```python
from build123d import *

# Parameters (mm, degrees)
F0_W      = 38.1
F0_H      = 38.1
F0_R      = 6.746875
F1_DEPTH  = 95.25
F3_D      = 4.0386
F3_DEPTH  = 12.7
F3_TIP    = 1.213317848
F5_D      = 4.0386
F5_DEPTH  = 12.7
F5_TIP    = 1.213317848
F6_R      = 9.525
F6_R_2    = 6.746875
F7_DEPTH  = 2.921
F8_R      = 9.525
F8_R_2    = 6.746875
F9_DEPTH  = 2.921
F11_D     = 8.45058
F11_DEPTH = 15.875
F11_TIP   = 2.538810365


with BuildPart() as f1:
    # F0 (on Front) → F1 (new body)
    with BuildSketch(Plane.XZ):
        Rectangle(F0_W, F0_H)
        Circle(F0_R, mode=Mode.SUBTRACT)
    extrude(amount=F1_DEPTH)

    # F3
    with Locations(Plane(origin=(0, 0, 0), x_dir=(-1, 0, 0), z_dir=(0, 1, 0))):
        with Locations((-12.7, -12.7), (-12.7, 12.7), (12.7, 12.7), (12.7, -12.7)):
            Hole(F3_D / 2, depth=F3_DEPTH)
            with Locations((0, 0, -(F3_DEPTH + F3_TIP / 2))):  # 118° drill point
                Cone(0, F3_D / 2, F3_TIP, mode=Mode.SUBTRACT)

    # F5
    with Locations(Plane.XZ.offset(95.25)):
        with Locations((-12.7, 12.7), (-12.7, -12.7), (12.7, -12.7), (12.7, 12.7)):
            Hole(F5_D / 2, depth=F5_DEPTH)
            with Locations((0, 0, -(F5_DEPTH + F5_TIP / 2))):  # 118° drill point
                Cone(0, F5_D / 2, F5_TIP, mode=Mode.SUBTRACT)

    # F6 (on face) → F7 (cut)
    with BuildSketch(Plane.XZ.offset(95.25)):
        Circle(F6_R)
        Circle(F6_R_2, mode=Mode.SUBTRACT)
    extrude(amount=-F7_DEPTH, mode=Mode.SUBTRACT)

    # F8 (on face) → F9 (cut)
    with BuildSketch(Plane(origin=(0, 0, 0), x_dir=(-1, 0, 0), z_dir=(0, 1, 0))):
        Circle(F8_R)
        Circle(F8_R_2, mode=Mode.SUBTRACT)
    extrude(amount=-F9_DEPTH, mode=Mode.SUBTRACT)

    # F11
    with Locations(Plane.YZ.offset(19.05)):
        with Locations((-47.625, 0)):
            Hole(F11_D / 2, depth=F11_DEPTH)
            with Locations((0, 0, -(F11_DEPTH + F11_TIP / 2))):  # 118° drill point
                Cone(0, F11_D / 2, F11_TIP, mode=Mode.SUBTRACT)


solid = f1.part
```
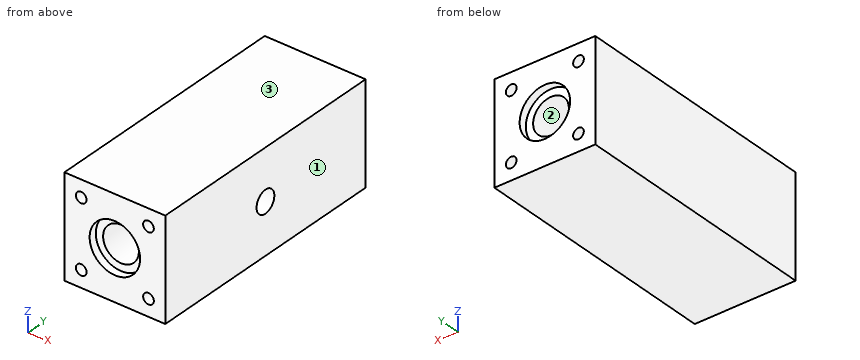
Verification items for the finished model (mm, model axes). Face numbers are marked on the shaded views. Round coordinates to 2 decimals unless told otherwise and drop trailing zeros. Write each loop counter-clockwise with the first axis right and the second up, starting at its lowest first coordinate (ties: lowest second). Pieces come first, ordered by that corner, then holes.
1. Section check C-C on y = -64. Enter the section's corners in (x, z), plus the area to 3 significant figures.
2. Gauge pin test, flat ends, axial feed: P1, Ø3.5, axis at x = 12.7, z = -12.7, coming from the -Y side; P2, Ø3, axis at x = -12.7, z = 12.7, coming from the +Y side; P3, Ø5.5, axis at x = 2.5, z = -4.5, coming from the +Y side; P4, Ø12, axis at x = 0, z = 0, coming from the +Y side. Record the tip position at first contact, or that the pin passes through.
3. Section check B-B on x = 0. Enter the section's corners in (y, z) (3 decimals), plus the area to 3 significant figures.
4. Draft check along X on the marked faces 1, 2 and 3. Enter one of: +X half, -X half, draft (parallel to the pull), parting line (faces both ways), or undercut.
5. Scan lines: L1, parallel to X at y = -2.25, z = 12.7; L2, parallel to Z at x = 0, y = -74. Record each from-to range of solid material in increasing order.
6. Section check A-A on z = 0. Enter the section's corners in (x, y) (3 decimals), plus the area to 3 significant figures.
Answer:
1. outline: (-19.05, -19.05) - (19.05, -19.05) - (19.05, 19.05) - (-19.05, 19.05) - close; hole circle Ø13.49 at (0, 0)
1. area: 1,310 mm2
2. P1: stops at y = -82.39
2. P2: stops at y = -13.01
2. P3: stops at y = -2.92
2. P4: passes through
3. outline: (-95.25, -19.05) - (0, -19.05) - (0, -9.525) - (-2.921, -9.525) - (-2.921, -6.747) - (-92.329, -6.747) - (-92.329, -9.525) - (-95.25, -9.525) - close; (-95.25, 9.525) - (-92.329, 9.525) - (-92.329, 6.747) - (-2.921, 6.747) - (-2.921, 9.525) - (0, 9.525) - (0, 19.05) - (-95.25, 19.05) - close
3. area: 2,310 mm2
4. face 1: +X half
4. face 2: undercut
4. face 3: draft
5. L1: x = -19.05 to -14.72, -10.68 to 10.68, 14.72 to 19.05
5. L2: z = -19.05 to -6.75, 6.75 to 19.05
6. outline: (-19.05, -95.25) - (-9.525, -95.25) - (-9.525, -92.329) - (-6.747, -92.329) - (-6.747, -2.921) - (-9.525, -2.921) - (-9.525, 0) - (-19.05, 0) - close; (6.747, -92.329) - (9.525, -92.329) - (9.525, -95.25) - (19.05, -95.25) - (19.05, -51.85) - (6.747, -51.85) - close; (6.747, -43.4) - (19.05, -43.4) - (19.05, 0) - (9.525, 0) - (9.525, -2.921) - (6.747, -2.921) - close
6. area: 2,210 mm2
